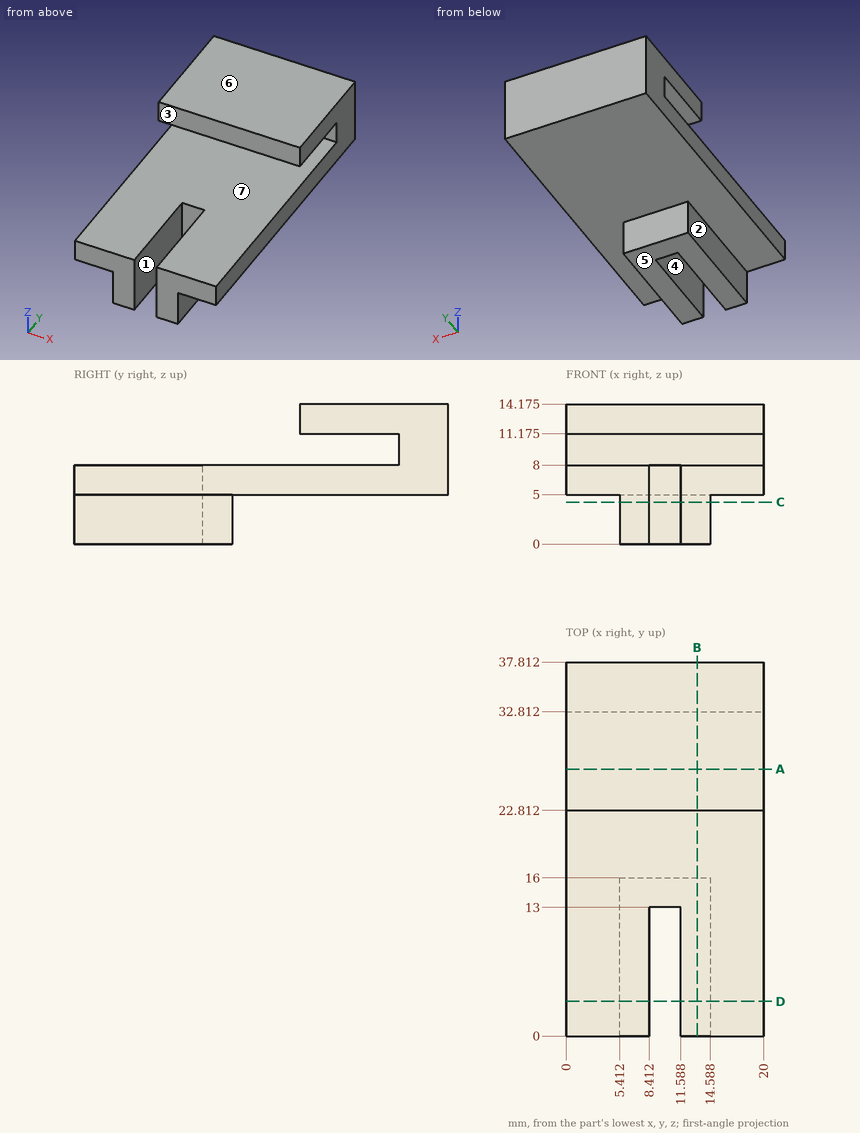
Design review of the part shown in the three views and the two pictorial views. Dimensions are in mm from the part's minimum x, y and z. A direction names the side the tool comes from. Coordinates: 2 decimals unless noted, no trailing zeros. Loops run counter-clockwise (first coordinate to the right, second up) from the corner with the lowest first, then second, coordinate; pieces in that order, holes last. Notation, with made-up numbers: (51.25, 85) -> (75.25, 85) arc R5 cw to (75.25, 91) -> close; hole circle Ø2 at (67.25, 55). An arc over 180 degrees is marked (long way). Answer as CSV lines item,"result".
Item 1: Draft analysis for pull direction Z (two halves, no side actions). For the marked faces 4, 5, 6 and 7, state which applies: +Z half, -Z half, draft (parallel to the pull), parting line (faces both ways), or undercut.
Results below:
face 4,"draft"
face 5,"-Z half"
face 6,"+Z half"
face 7,"undercut"
Item 2: For L1, parallel to Z at x = 9.25, y = 23 (1 decimal); L2, parallel to X at y = 2.5, z = 1.5; L3, parallel to Z at x = 6.5, y = 22, list the stretches that pass through material, from the lowest coordinate up.
Results below:
L1,"z = 5 to 8, 11.2 to 14.2"
L2,"x = 5.41 to 8.41, 11.59 to 14.59"
L3,"z = 5 to 8"
Item 3: Take a section at B-B, the plane x = 13.25. State the section outline as (y, z) points (1 decimal).
Results below:
outline,"(0, 0) -> (16, 0) -> (16, 5) -> (37.8, 5) -> (37.8, 14.2) -> (22.8, 14.2) -> (22.8, 11.2) -> (32.8, 11.2) -> (32.8, 8) -> (0, 8) -> close"
Item 4: Take a section at A-A, the plane y = 27. State the section outline as (x, z) points (1 decimal).
Results below:
outline,"(0, 5) -> (20, 5) -> (20, 8) -> (0, 8) -> close; (0, 11.2) -> (20, 11.2) -> (20, 14.2) -> (0, 14.2) -> close"
Item 5: Take a section at D-D, the plane y = 3.5. State the section outline as (x, z) points.
Results below:
outline,"(0, 5) -> (5.41, 5) -> (5.41, 0) -> (8.41, 0) -> (8.41, 8) -> (0, 8) -> close; (11.59, 0) -> (14.59, 0) -> (14.59, 5) -> (20, 5) -> (20, 8) -> (11.59, 8) -> close"
Item 6: Insertion check: pin 1 (1.6 mm diameter, centred on x = 9.5, z = 2.5, fed in from -Y); pin 2 (1.5 mm diameter, centred on y = 4.5, z = 1.5, fed in from -X); pin 3 (8 mm diameter, centred on x = 11, y = 4.5, fed in from +Z). Each pin has a flat end and moves straight along its axis. Give the tip position at first contact, or say it passes through.
Results below:
pin 1,"stops at y = 13"
pin 2,"stops at x = 5.41"
pin 3,"stops at z = 8"
Item 7: Machinability: for the marked faces 1, 2 and 3, which of the approach directions +Z, -Z, +X, -X, +Y, -Y give a long, thin tool a straight path to every point of the face, cutting with its end or side? Answer none if there is none.
Results below:
face 1,"+Z, -Z, -Y"
face 2,"-Z, -X, +Y, -Y"
face 3,"+Z, +X, -X, -Y"
Item 8: Take a section at C-C, the plane z = 4.25. State the section outline as (x, y) points.
Results below:
outline,"(5.41, 0) -> (8.41, 0) -> (8.41, 13) -> (11.59, 13) -> (11.59, 0) -> (14.59, 0) -> (14.59, 16) -> (5.41, 16) -> close"
